Geometry check sheet. Reference: the model listing, model coordinates, mm. Round coordinates to 2 decimals unless told otherwise and drop trailing zeros. Write each loop counter-clockwise with the first axis right and the second up, starting at its lowest first coordinate (ties: lowest second). Pieces come first, ordered by that corner, then holes. Notation, with made-up numbers: (60, 59) - (95, 59) arc R31 ccw to (95, 90) - close; hole circle Ø10 at (30.5, -20). An arc over 180 degrees is marked (long way). Return JSON: item names as keys, results as strings.
Autodesk Inventor part; units mm, degrees
ref_plane "YZ Plane" through (0, 0, 0) normal (1, 0, 0) x (0, 1, 0)
ref_plane "XZ Plane" through (0, 0, 0) normal (0, 1, 0) x (-1, 0, 0)
ref_plane "XY Plane" through (0, 0, 0) normal (0, 0, 1) x (1, 0, 0)
sketch "Sketch1" plane through (0, 0, 0) normal (0, 0, 1) x (1, 0, 0)
  line L0 (0, 0) -> (80, 0)
  line L1 (80, 0) -> (80, 13)
  line L2 (80, 13) -> (0, 13)
  line L3 (0, 13) -> (0, 0)
  dimension "d0" = 80
  dimension "d1" = 13
extrude "Extrusion1" add sketch "Sketch1" along normal blind 13
sketch "Sketch2" plane through (0, 0, 13) normal (0, 0, 1) x (1, 0, 0)
  circle A0 centre (35.7535, 6.5) radius 5.5
  circle A1 centre (43.7535, 6.4786) radius 5.5
  line L0 (80, 13) -> (0, 13)
  line L1 (80, 0) -> (80, 13)
  line L2 (0, 13) -> (0, 0)
  line L3 (80, 0) -> (80, 13)
  line L4 (80, 13) -> (0, 13)
  line L5 (0, 13) -> (0, 0)
  line L6 (0, 0) -> (80, 0)
  point P0 (39.7636, 10.2642)
  point P1 (39.7434, 2.7144)
  point P2 (40, 13)
  dimension "d14" = 13
  dimension "d15" = 80
  dimension "d17" = 40
  dimension "d18" = 19
  dimension "d19" = 6.5
  dimension "d20" = 8
extrude "Extrusion2" cut sketch "Sketch2" against normal blind 13 contours A0 A1 | A0 A1 | A1 A0
properties part number "Weight_Sensor"
(1) Section check B-B, the plane x = 35. Enter the section's corners in (y, z), plus the area to 3 significant figures.
Response values:
{"outline": "(0, 0) - (1.05, 0) - (1.05, 13) - (0, 13) - close; (11.95, 0) - (13, 0) - (13, 13) - (11.95, 13) - close", "area": "27.3 mm^2"}
(2) Section check A-A, the plane y = 8. Enter the section's corners in (x, z), plus the area to 4 significant figures.
Response values:
{"outline": "(0, 0) - (30.46, 0) - (30.46, 13) - (0, 13) - close; (49.04, 0) - (80, 0) - (80, 13) - (49.04, 13) - close", "area": "798.5 mm^2"}
(3) Release check for a two-part mould opening along X. For faces 1 (the face through (39.4, 10.9, 13)), 2 (the face through (30.257, 6.698, 6.591)), 3 (the face through (49.25, 6.28, 6.59)), 4 (the face through (0, 7, 6)) record: pulls with the +X half, pulls with the -X half, needs draft (parallel to the pull), parting line crosses it, or undercut.
Response values:
{"face 1": "needs draft", "face 2": "undercut", "face 3": "undercut", "face 4": "pulls with the -X half"}
(4) Material ranges on line 1 along X through (y, z) = (11.5, 11.5); line 2 along X through (y, z) = (6.5, 6.5); line 3 along Y through (x, z) = (36, 10), recorded low to high. Write a range as [from, to].
Response values:
{"line 1": "x = [0, 33.46], [38.04, 41.51], [46, 80]", "line 2": "x = [0, 30.25], [49.25, 80]", "line 3": "y = [0, 1.01], [11.99, 13]"}
(5) Section check C-C, the plane z = 8.5. Enter the section's corners in (x, y), plus the area to 4 significant figures.
Response values:
{"outline": "(0, 0) - (80, 0) - (80, 13) - (0, 13) - close; hole (39.74, 2.71) arc R5.5 ccw (long way) to (39.76, 10.26) arc R5.5 ccw (long way) to start", "area": "865.5 mm^2"}
